Read the model definition and answer for the solid it produces. Units are mm, in the model's axes. A direction names the side the tool comes from. Coordinates: 2 decimals unless noted, no trailing zeros. Order: outer loops, then holes, each group sorted by start corner. A loop starts at its lowest first (then second) coordinate and runs counter-clockwise, first axis right, second up. Notation, with made-up numbers: (-23, 64.25) -> (8, 64.25) arc R33 cw to (8, 93.25) -> close; hole circle Ø1 at (23.25, -12). An arc over 180 degrees is marked (long way). Answer as a JSON object with one key per item and string values. Group by question number.
1) Consider L1, parallel to X at y = 81, z = 25.5; L2, parallel to Z at x = 13, y = 34.5; L3, parallel to Y at x = 15, z = 28. Determine where each line is inside the solid, lowest interval first.
2) A tool of negligible diameter and unlimited length cuts with its end or side. For faces 1 (the flat face through (42, 60, 70)), 2 (the cylindrical face through (84, 32, 22)), 3 (the cylindrical face through (47.45, 54.1, 18.86)), 4 (the flat face through (48, 38, 22)), 5 (the flat face through (47, 41, 23)), from which of +Z, -Z, +X, -X, +Y, -Y can it reach the whole face along a straight path? Write none if from no direction.
3) Determine the mould class of faces 6 (the flat face through (47, 0, 9)), 7 (the flat face through (42, 64, 64)), 8 (the flat face through (49, 55, 25)), 9 (the cylindrical face through (47.5, 54.1, 31.14)) for opening direction Z: released by +Z, released by -Z, zero draft, split by the parting line, or undercut.
4) Given pin 1 (8 mm diameter, centred on x = 44.5, y = 31, fed in from +Z); pin 2 (6 mm diameter, centred on y = 54.5, z = 51, fed in from +X); pin 3 (10 mm diameter, centred on x = 21, y = 14.5, fed in from -Z); pin 4 (16 mm diameter, centred on x = 50, y = 32, fed in from -Z), each flat-ended and moving along its own axis, determine where each tip first touches the part or whether it passes through.
5) Section A-A on y = 50 is taken. Determine the outline of the cut face in (x, z).
from build123d import *

# Parameters (mm, degrees)
F0_W      = 96
F0_H      = 90
F1_DEPTH  = 18
F2_W      = 72
F2_H      = 38
F4_DEPTH  = 58
F6_DEPTH  = 38
F7_W      = 8
F7_H      = 12
F8_DEPTH  = 60.001
F10_DEPTH = 72.001
F11_W     = 20
F11_H     = 5
F12_DEPTH = 96
F13_W     = 46
F13_H     = 26
F14_DEPTH = 5
F15_W     = 46
F15_H     = 12
F17_DEPTH = 3
F18_W     = 3
F18_H     = 14
F19_DEPTH = 72
F20_R     = 2.99999


# Not quite as in the source:
# - a fillet or chamfer is up to 0.001 mm smaller than in the source, because OpenCascade refuses the exact size


with BuildPart() as f1:
    # F0 (on Top) → F1 (new body)
    with BuildSketch(Plane.XY):
        with Locations((48, 45)):
            Rectangle(F0_W, F0_H)
    extrude(amount=F1_DEPTH)

    # F2 (on face) → F4 (join, through all)
    with BuildSketch(Plane.XY.offset(18)):
        with Locations((48, 71)):
            Rectangle(F2_W, F2_H)
    extrude(amount=F4_DEPTH)

    # F5 (on face) → F6 (cut, through all)
    with BuildSketch(Plane.XZ.offset(-52)):
        Polygon((84, 52), (84, 76), (60, 76), align=None)
    extrude(amount=-F6_DEPTH, mode=Mode.SUBTRACT)

    # F7 (on face) → F8 (cut, through all)
    with BuildSketch(Plane(origin=(12, 0, 0), x_dir=(0, -1, 0), z_dir=(-1, 0, 0))):
        with Locations((-64, 70)):
            Rectangle(F7_W, F7_H)
    extrude(amount=-F8_DEPTH, mode=Mode.SUBTRACT)

    # F9 (on face) → F10 (cut, through all)
    with BuildSketch(Plane(origin=(12, 0, 0), x_dir=(0, -1, 0), z_dir=(-1, 0, 0))):
        Polygon((-90, 40), (-76, 76), (-90, 76), align=None)
    extrude(amount=-F10_DEPTH, mode=Mode.SUBTRACT)

    # F11 (on face) → F12 (cut, through all)
    with BuildSketch(Plane.YZ.offset(96)):
        with Locations((32, 2.5)):
            Rectangle(F11_W, F11_H)
    extrude(amount=-F12_DEPTH, mode=Mode.SUBTRACT)

    # F13 (on face) → F14 (join)
    with BuildSketch(Plane.XY.offset(18)):
        with Locations((48, 31.9999999999)):
            Rectangle(F13_W, F13_H)
        with BuildLine():
            Line((25, 18.9999999999), (25, 44.9999999999))
            ThreePointArc((25, 44.9999999999), (12, 31.9999999999), (25, 18.9999999999))
        make_face()
        with BuildLine():
            ThreePointArc((71, 18.9999999999), (84, 31.9999999999), (71, 44.9999999999))
            Line((71, 44.9999999999), (71, 18.9999999999))
        make_face()
    extrude(amount=F14_DEPTH)

    # F15 (on face) → F17 (cut, through all)
    with BuildSketch(Plane.XY.offset(23)):
        with Locations((48, 31.9999999999)):
            Rectangle(F15_W, F15_H)
        with BuildLine():
            Line((25, 25.9999999999), (25, 37.9999999999))
            ThreePointArc((25, 37.9999999999), (19, 31.9999999999), (25, 25.9999999999))
        make_face()
        with BuildLine():
            ThreePointArc((71, 25.9999999999), (77, 31.9999999999), (71, 37.9999999999))
            Line((71, 37.9999999999), (71, 25.9999999999))
        make_face()
    extrude(amount=-F17_DEPTH, mode=Mode.SUBTRACT)

    # F18 (on face) → F19 (cut, through all)
    with BuildSketch(Plane.YZ.offset(84)):
        with Locations((53.5, 25)):
            Rectangle(F18_W, F18_H)
    extrude(amount=-F19_DEPTH, mode=Mode.SUBTRACT)

    # F20 (radius 3 in the source; OpenCascade refuses exactly that, so slightly less here)
    f20_edges = [f1.edges().sort_by_distance(p)[0] for p in [
        (48, 19, 18),
        (48, 55, 18),
        (48, 55, 32),
        (84, 72.5, 18),
        (12, 72.5, 18),
        (0, 45, 18),
        (96, 45, 18),
        (96, 0, 9),
        (0, 0, 9),
        (0, 90, 9),
        (96, 90, 9),
    ]]
    fillet(f20_edges, radius=F20_R)


solid = f1.part
Worked answers:
{
 "1": {"L1": "x = 12 to 84", "L2": "z = 5 to 23", "L3": "y = 55 to 90"},
 "2": {"face 1": "+Z, +X, -X", "face 2": "+Z, +X", "face 3": "+X, -X", "face 4": "+Z", "face 5": "+Z, +X, -X, -Y"},
 "3": {"face 6": "zero draft", "face 7": "released by +Z", "face 8": "undercut", "face 9": "undercut"},
 "4": {"pin 1": "stops at z = 20", "pin 2": "stops at x = 84", "pin 3": "stops at z = 0", "pin 4": "stops at z = 5"},
 "5": {"outline": "(0, 0) -> (96, 0) -> (96, 15) arc R3 ccw to (93, 18) -> (3, 18) arc R3 ccw to (0, 15) -> close"}
}
